Source: CAD feature listing. Evaluate the final solid. Frame: model axes, mm. A direction names the side the tool comes from. Round coordinates to 2 decimals unless told otherwise and drop trailing zeros. Loops run counter-clockwise (first coordinate to the right, second up) from the corner with the lowest first, then second, coordinate; pieces in that order, holes last. Notation, with made-up numbers: (17, 40) -> (67, 40) arc R33 ccw to (67, 75) -> close; hole circle Ø11 at (-2, 22.25). An arc over 180 degrees is marked (long way). Return JSON: item names as keys, results as strings. Group by question number.
```python
from build123d import *

# Parameters (mm, degrees)
F1_DEPTH = 8
F2_DEPTH = 3
F3_DEPTH = 8


with BuildPart() as f1:
    # F0 (on Front) → F1 (new body)
    with BuildSketch(Plane.XZ):
        with BuildLine():
            ThreePointArc((4.330127, 2.5), (4.829629, 1.294095), (5, 0))
            ThreePointArc((5, 0), (-1.294095, -4.829629), (-4.330127, 2.5))
            ThreePointArc((-4.330127, 2.5), (-4.769358, 4.13923), (-6.408588, 3.7))
            ThreePointArc((-6.408588, 3.7), (-7.31394, -1.125289), (-5, -5.455273))
            ThreePointArc((-5, -5.455273), (-3.234602, -6.655625), (-1.2, -7.302055))
            ThreePointArc((-1.2, -7.302055), (0, -7.4), (1.2, -7.302055))
            ThreePointArc((1.2, -7.302055), (3.234602, -6.655625), (5, -5.455273))
            ThreePointArc((5, -5.455273), (6.773478, -2.979933), (7.4, 0))
            ThreePointArc((7.4, 0), (7.147851, 1.915261), (6.408588, 3.7))
            ThreePointArc((6.408588, 3.7), (4.769358, 4.13923), (4.330127, 2.5))
        make_face()
    extrude(amount=F1_DEPTH)

    # F0 (on Front) → F2 (join)
    with BuildSketch(Plane.XZ):
        with BuildLine():
            ThreePointArc((-1.2, -7.302055), (-3.234602, -6.655625), (-5, -5.455273))
            Line((-5, -5.455273), (-5, -65.455273))
            Line((-5, -65.455273), (-1.2, -69.255273))
            Line((-1.2, -69.255273), (-1.2, -7.302055))
        make_face()
        with BuildLine():
            Line((5, -65.455273), (5, -5.455273))
            ThreePointArc((5, -5.455273), (3.234602, -6.655625), (1.2, -7.302055))
            Line((1.2, -7.302055), (1.2, -69.255273))
            Line((1.2, -69.255273), (5, -65.455273))
        make_face()
        with BuildLine():
            ThreePointArc((1.2, -7.302055), (0, -7.4), (-1.2, -7.302055))
            Line((-1.2, -7.302055), (-1.2, -69.255273))
            Line((-1.2, -69.255273), (0, -70.455273))
            Line((0, -70.455273), (1.2, -69.255273))
            Line((1.2, -69.255273), (1.2, -7.302055))
        make_face()
    extrude(amount=F2_DEPTH)

    # F0 (on Front) → F3 (join)
    with BuildSketch(Plane.XZ):
        with BuildLine():
            ThreePointArc((1.2, -7.302055), (0, -7.4), (-1.2, -7.302055))
            Line((-1.2, -7.302055), (-1.2, -69.255273))
            Line((-1.2, -69.255273), (0, -70.455273))
            Line((0, -70.455273), (1.2, -69.255273))
            Line((1.2, -69.255273), (1.2, -7.302055))
        make_face()
    extrude(amount=F3_DEPTH)


solid = f1.part
```
(1) Cut plane C-C (x = -3.5). Return loops of the section in (y, z).
(2) Pin query (flat end, axial travel): pin 1 (2 mm diameter, centred on x = 1.5, y = -5.5, fed in from +Z); pin 2 (4 mm diameter, centred on y = -4.5, z = -6.5, fed in from -X); pin 3 (1.9 mm diameter, centred on x = 3, z = -42.5, fed in from -Y). Return the tip coordinate at first contact, or that it passes through.
(3) Set-up query: faces 1 (the face through (5, -1, -36)), 2 (the face through (-1.2, -5, -38)), 3 (the face through (-5, -1, -35)), 4 (the face through (3.208, -5.465, -6.669)). Return all of +Z, -Z, +X, -X, +Y, -Y with unobstructed straight access to the full face (end or side cutting, diameter ignored); none if empty.
(4) Cut plane A-A (x = 2.5). Return loops of the section in (y, z).
(5) Cut plane B-B (y = -6). Return loops of the section in (x, z), and give its area (3 significant figures).
(6) Cut plane D-D (y = -2.25). Return loops of the section in (x, z), and give its area (3 significant figures).
(7) Mould query, pull axis X, two halves, no side actions, for faces 5 (the face through (-4.75, -3.94, 4.13)), 6 (the face through (4.79, -3.94, 4.15)), 7 (the face through (1.909, -2.166, -68.546)), 8 (the face through (-3.262, -5.465, -6.642)). Classes: released by +X, released by -X, zero draft, split by the parting line, or undercut.
(8) Ray query, line 1 (X direction, y = -2, z = 0); line 2 (X direction, y = -1.5, z = -56); line 3 (Y direction, x = 1.75, z = -13.5). Return the intervals inside material, ascending.
Answers follow:
{
 "1": {"outline": "(-8, -6.52) -> (-3, -6.52) -> (-3, -66.96) -> (0, -66.96) -> (0, -3.57) -> (-8, -3.57) -> close"},
 "2": {"pin 1": "z = -4.33", "pin 2": "x = -5.87", "pin 3": "y = -3"},
 "3": {"face 1": "-Z, +X, +Y, -Y", "face 2": "-Z, -X, -Y", "face 3": "-Z, -X, +Y, -Y", "face 4": "-Z, +X, -Y"},
 "4": {"outline": "(-8, -6.96) -> (-3, -6.96) -> (-3, -67.96) -> (0, -67.96) -> (0, -4.33) -> (-8, -4.33) -> close"},
 "5": {"outline": "(-6.41, 3.7) arc R7.4 ccw to (-5, -5.46) arc R7.4 ccw to (-1.2, -7.3) -> (-1.2, -69.26) -> (0, -70.46) -> (1.2, -69.26) -> (1.2, -7.3) arc R7.4 ccw to (5, -5.46) arc R7.4 ccw to (7.4, 0) arc R7.4 ccw to (6.41, 3.7) arc R1.2 ccw to (4.33, 2.5) arc R5 cw to (5, 0) arc R5 cw (long way) to (-4.33, 2.5) arc R1.2 ccw to start", "area": "217 mm^2"},
 "6": {"outline": "(-6.41, 3.7) arc R7.4 ccw to (-5, -5.46) -> (-5, -65.46) -> (0, -70.46) -> (5, -65.46) -> (5, -5.46) arc R7.4 ccw to (7.4, 0) arc R7.4 ccw to (6.41, 3.7) arc R1.2 ccw to (4.33, 2.5) arc R5 cw to (5, 0) arc R5 cw (long way) to (-4.33, 2.5) arc R1.2 ccw to start", "area": "679 mm^2"},
 "7": {"face 5": "undercut", "face 6": "undercut", "face 7": "released by +X", "face 8": "released by -X"},
 "8": {"line 1": "-7.4 to -5, 5 to 7.4", "line 2": "-5 to 5", "line 3": "-3 to 0"}
}
